Here's how the part is built. I have some questions about the finished solid (model axes, mm). Face numbers are marked on the shaded views. A direction names the side the tool comes from. Round coordinates to 2 decimals unless told otherwise and drop trailing zeros. Order: outer loops, then holes, each group sorted by start corner. A loop starts at its lowest first (then second) coordinate and runs counter-clockwise, first axis right, second up. Notation, with made-up numbers: M 67,-13 L 81,-13 A31 ccw 81,11 Z; hole C 56.25,15 d10. An arc over 180 degrees is marked long. Write item = value, one per line. Start each with the question number.
Item 1: I want a section at C-C, the plane y = 43. List the corners of the cut face in (x, z) for me.
Item 2: I want a section at B-B, the plane x = -3.25. List the corners of the cut face in (y, z) for me.
Item 3: I want a section at D-D, the plane z = -2.25. List the corners of the cut face in (x, y) for me.
Item 4: I want a section at A-A, the plane z = 0. List the corners of the cut face in (x, y) for me, plus the area to 3 significant figures.
Item 5: I'm going to push flat-ended pins straight in: P1, Ø6, axis at x = 0, z = 5.5, coming from the -Y side; P2, Ø4, axis at y = 37, z = 6.5, coming from the +X side; P3, Ø4, axis at x = 2, y = 12.5, coming from the +Z side; P4, Ø6, axis at x = -3.5, y = 6, coming from the -Z side. Where does each tip first touch, or does it pass through?
Item 6: For the marked faces 1 and 2, which set-ups out of +Z, -Z, +X, -X, +Y, -Y let a thin tool reach every point of the face, with its end or its side?
Item 7: Please list where these lines run through material, in increasing order: L1, parallel to Y at x = 1.75, z = 4.5; L2, parallel to Y at x = 2, z = -7; L3, parallel to Z at x = -0.25, y = 21.5.
```python
from build123d import *

# Parameters (mm, degrees)
SKETCH_1_R          = 4
EXTRUDE_1_DEPTH     = 59.9
SKETCH_1_3_R        = 5
SKETCH_1_3_R_2      = 4
EXTRUDE_2_DEPTH     = 46.7
SKETCH_1_4_R        = 7.9
SKETCH_1_4_R_2      = 5
EXTRUDE_3_DEPTH     = 6.7
CUT_EXTRUDE_1_DEPTH = 3


with BuildPart() as part:
    # Sketch 1 → Extrude 1 (new body)
    with BuildSketch(Plane(origin=(0, 0, 0), x_dir=(1, 0, 0), z_dir=(0, 1, 0))):
        with Locations(Location((0, 0, 0), (0, 0, 270))):
            Circle(SKETCH_1_R)
    extrude(amount=EXTRUDE_1_DEPTH)

    # Sketch 1_3 → Extrude 2 (add)
    with BuildSketch(Plane(origin=(0, 0, 0), x_dir=(1, 0, 0), z_dir=(0, 1, 0))):
        with Locations(Location((0, 0, 0), (0, 0, 270))):
            Circle(SKETCH_1_3_R)
        with Locations(Location((0, 0, 0), (0, 0, 270))):
            Circle(SKETCH_1_3_R_2, mode=Mode.SUBTRACT)
    extrude(amount=EXTRUDE_2_DEPTH)

    # Sketch 1_4 → Extrude 3 (add)
    with BuildSketch(Plane(origin=(0, 0, 0), x_dir=(1, 0, 0), z_dir=(0, 1, 0))):
        with Locations(Location((0, 0, 0), (0, 0, 270))):
            Circle(SKETCH_1_4_R)
        with Locations(Location((0, 0, 0), (0, 0, 270))):
            Circle(SKETCH_1_4_R_2, mode=Mode.SUBTRACT)
    extrude(amount=EXTRUDE_3_DEPTH)

    # Sketch 2 → Cut-Extrude 1 (cut)
    with BuildSketch(Plane.XZ):
        Polygon((2.5, 1.443375673), (0, 2.886751346), (-2.5, 1.443375673), (-2.5, -1.443375673), (0, -2.886751346), (2.5, -1.443375673), align=None)
    extrude(amount=-CUT_EXTRUDE_1_DEPTH, mode=Mode.SUBTRACT)


solid = part.part
```
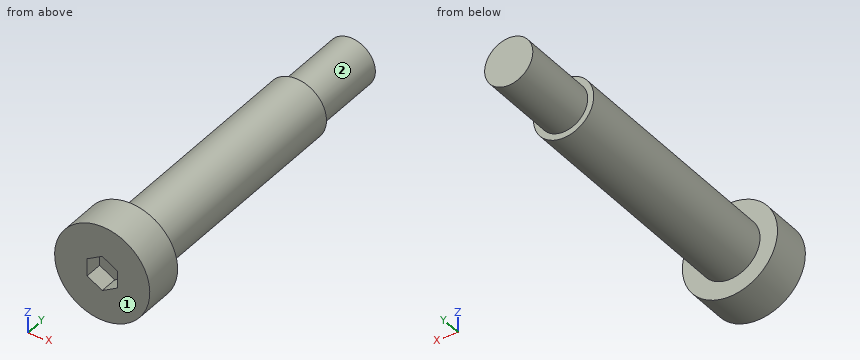
Filled in:
q1.outline = C 0,0 d10
q2.outline = M 0,-7.2 L 6.7,-7.2 L 6.7,-3.8 L 46.7,-3.8 L 46.7,-2.33 L 59.9,-2.33 L 59.9,2.33 L 46.7,2.33 L 46.7,3.8 L 6.7,3.8 L 6.7,7.2 L 0,7.2 Z
q3.outline = M -7.57,0 L -1.1,0 L -1.1,3 L 1.1,3 L 1.1,0 L 7.57,0 L 7.57,6.7 L 4.47,6.7 L 4.47,46.7 L 3.31,46.7 L 3.31,59.9 L -3.31,59.9 L -3.31,46.7 L -4.47,46.7 L -4.47,6.7 L -7.57,6.7 Z
q4.outline = M -7.9,0 L -2.5,0 L -2.5,3 L 2.5,3 L 2.5,0 L 7.9,0 L 7.9,6.7 L 5,6.7 L 5,46.7 L 4,46.7 L 4,59.9 L -4,59.9 L -4,46.7 L -5,46.7 L -5,6.7 L -7.9,6.7 Z
q4.area = 596 mm^2
q5.P1 = 0
q5.P2 = 2.18
q5.P3 = 5
q5.P4 = -7.88
q6.face_1 = +Z, -Z, +X, -X, -Y
q6.face_2 = +Y
q7.L1 = 0 to 46.7
q7.L2 = 0 to 6.7
q7.L3 = -4.99 to 4.99
